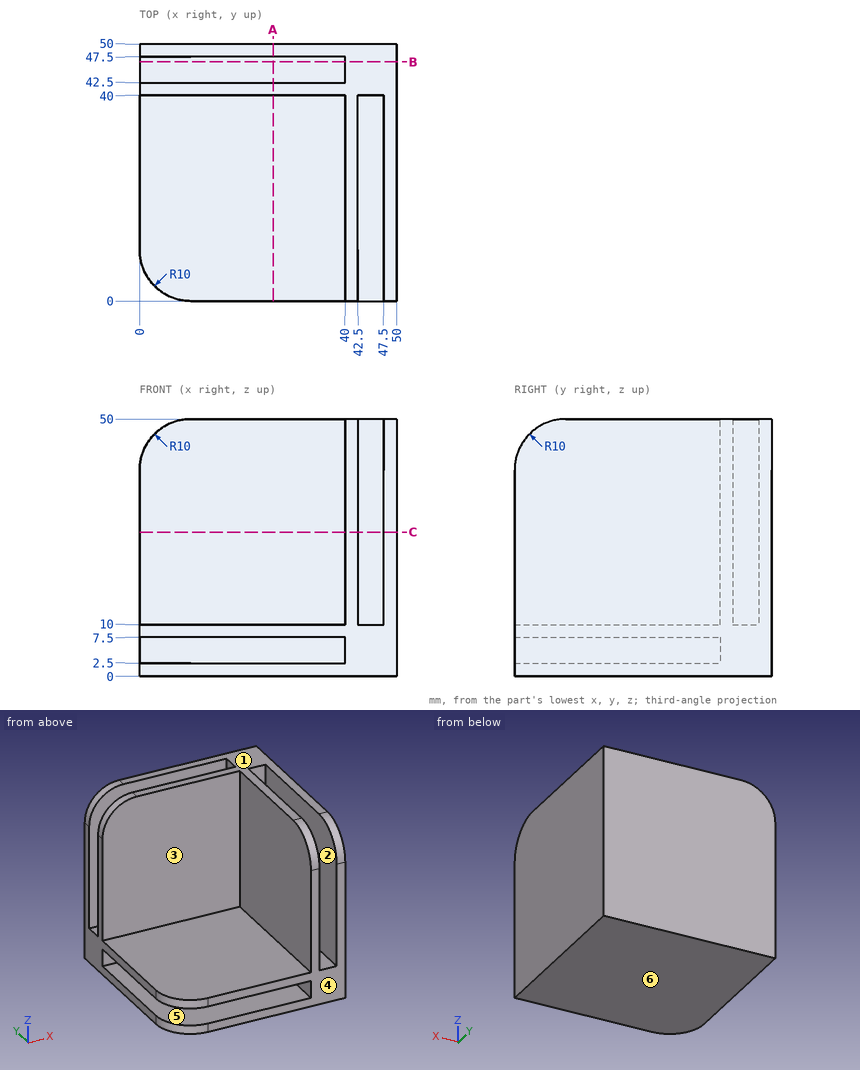
Could you check a few things on this drawing? It's one solid part, dimensions in mm from its lowest x, y, z. A direction names the side the tool comes from. Give positions to 0.01 mm unless a question says otherwise; leave off trailing zeros. Order: outer loops, then holes, each group sorted by start corner. A loop starts at its lowest first (then second) coordinate and runs counter-clockwise, first axis right, second up.
1. Thinking about a two-plate mould opening in Z: for the marked faces 4, 5 and 6, which applies, +Z half, -Z half, draft (parallel to the pull), parting line (faces both ways), or undercut?
Answers below:
face 4: draft
face 5: undercut
face 6: -Z half
2. For pin 1 (20 mm diameter, centred on x = 10.5, z = 25, fed in from -Y); pin 2 (20 mm diameter, centred on y = 13.5, z = 31.5, fed in from -X); pin 3 (1.5 mm diameter, centred on x = 29, y = 5.5, fed in from -Z); pin 4 (1.5 mm diameter, centred on x = 15.5, y = 45.5, fed in from +Z), each with a flat end and sliding along its axis, tell me the tip position at first contact or that it passes through.
Answers below:
pin 1: stops at y = 40
pin 2: stops at x = 40
pin 3: stops at z = 0
pin 4: stops at z = 10
3. I need wall thicknesses on L1, parallel to Z at x = 16, y = 6; L2, parallel to Y at x = 23, z = 25. Which ranges of each line are inside material? Lowest first, please.
Answers below:
L1: z = 0 to 2.5, 7.5 to 10
L2: y = 40 to 42.5, 47.5 to 50
4. Suppose I cut it at C-C (z = 28). Write out the boundary of the cut face in (x, y).
Answers below:
outline: (0, 40) - (40, 40) - (40, 0) - (42.5, 0) - (42.5, 40) - (47.5, 40) - (47.5, 0) - (50, 0) - (50, 50) - (0, 50) - (0, 47.5) - (40, 47.5) - (40, 42.5) - (0, 42.5) - close
5. Suppose I cut it at A-A (x = 26). Write out the boundary of the cut face in (y, z), plus the area to 3 significant figures.
Answers below:
outline: (0, 0) - (50, 0) - (50, 50) - (47.5, 50) - (47.5, 10) - (42.5, 10) - (42.5, 50) - (40, 50) - (40, 10) - (0, 10) - (0, 7.5) - (40, 7.5) - (40, 2.5) - (0, 2.5) - close
area: 500 mm2
6. Which directions (+Z, -Z, +X, -X, +Y, -Y) give clear straight access to the entire face, cutting with the end or side of a thin tool? Please do the marked faces 1, 2 and 3.
Answers below:
face 1: +Z, +X, -X, +Y, -Y
face 2: +Z, -Y
face 3: +Z, -X, -Y
7. Suppose I cut it at B-B (y = 46.5). Write out the boundary of the cut face in (x, z), plus the area to 3 significant figures.
Answers below:
outline: (0, 0) - (50, 0) - (50, 50) - (40, 50) - (40, 10) - (0, 10) - close
area: 900 mm2
